```python
from build123d import *

# Parameters (mm, degrees)
F1_DEPTH = 5
F2_COUNT = 3
F3_DEPTH = 5


with BuildPart() as f1:
    # F0 (on Top) → F1 (new body)
    with BuildSketch(Plane.XY):
        with BuildLine():
            ThreePointArc((-5.4248477433, 6.6765403938), (0, 8.602625452), (5.4248477433, 6.6765403938))
            Line((5.4248477433, 6.6765403938), (1.3544146049, 29.8043473585))
            Line((1.3544146049, 29.8043473585), (-1.3544146049, 29.8043473585))
            Line((-1.3544146049, 29.8043473585), (-5.4248477433, 6.6765403938))
        make_face()
        with BuildLine():
            ThreePointArc((-6.4909440333, -0.3429949805), (-6.4880250922, 0.3943734303), (-6.4016109203, 1.1266665987))
            Line((-6.4016109203, 1.1266665987), (-6.5999012756, 0))
            Line((-6.5999012756, 0), (-6.4909440333, -0.3429949805))
        make_face()
        with BuildLine():
            ThreePointArc((-6.4016109203, 1.1266665987), (3.01e-08, 6.5), (6.4016109308, 1.1266665393))
            Line((6.4016109308, 1.1266665393), (5.4248477433, 6.6765403938))
            ThreePointArc((5.4248477433, 6.6765403938), (0, 8.602625452), (-5.4248477433, 6.6765403938))
            Line((-5.4248477433, 6.6765403938), (-6.4016109203, 1.1266665987))
        make_face()
        with BuildLine():
            ThreePointArc((5.4826146341, -20.6491084281), (3.2218551697, -19.3014479363), (0.6594098664, -18.7005351105))
            Line((0.6594098664, -18.7005351105), (0, -20.7763427347))
            Line((0, -20.7763427347), (-0.6594098664, -18.7005351105))
            ThreePointArc((-0.6594098664, -18.7005351105), (-3.2230425543, -19.3019277422), (-5.4845879123, -20.6507413875))
            Line((-5.4845879123, -20.6507413875), (-6.6083723171, -21.7710077677))
            ThreePointArc((-6.6083723171, -21.7710077677), (-8.5655271696, -26.4946509242), (-7.4957432876, -31.494533146))
            Line((-7.4957432876, -31.494533146), (-7.1801960351, -32.0117500748))
            ThreePointArc((-7.1801960351, -32.0117500748), (-4.7747668767, -34.4304254189), (-1.6183226323, -35.7238470784))
            ThreePointArc((-1.6183226323, -35.7238470784), (0, -35.7604840323), (1.6183226323, -35.7238470784))
            ThreePointArc((1.6183226323, -35.7238470784), (4.7779827917, -34.4282780127), (7.1844511071, -32.0052918853))
            Line((7.1844511071, -32.0052918853), (7.4957432876, -31.494533146))
            ThreePointArc((7.4957432876, -31.494533146), (8.3201892844, -29.4566518987), (8.6011218908, -27.2763427347))
            ThreePointArc((8.6011218908, -27.2763427347), (8.0881303689, -24.3503480465), (6.6103478907, -21.7733800287))
            Line((6.6103478907, -21.7733800287), (5.4826146341, -20.6491084281))
        make_face()
        with BuildLine():
            ThreePointArc((6.5, -27.2763427347), (-4.5961940777, -31.8725368124), (0, -20.7763427347))
            ThreePointArc((0, -20.7763427347), (4.5961940777, -22.680148657), (6.5, -27.2763427347))
        make_face(mode=Mode.SUBTRACT)
        with BuildLine():
            ThreePointArc((1.6183226323, -35.7238470784), (0, -35.7604840323), (-1.6183226323, -35.7238470784))
            ThreePointArc((-1.6183226323, -35.7238470784), (0, -35.8774646255), (1.6183226323, -35.7238470784))
        make_face()
        with BuildLine():
            Line((1.3493711691, -16.5285522429), (4.2182307974, -7.4974458056))
            ThreePointArc((4.2182307974, -7.4974458056), (0, -8.602625452), (-4.2182307974, -7.4974458056))
            Line((-4.2182307974, -7.4974458056), (-1.3493910102, -16.5284897836))
            Line((-1.3493910102, -16.5284897836), (0, -15.183323063))
            Line((0, -15.183323063), (1.3493711691, -16.5285522429))
        make_face()
        with BuildLine():
            Line((5.4248477433, 6.6765403938), (6.4016109308, 1.1266665393))
            Line((6.4016109308, 1.1266665393), (6.5999012756, 0))
            Line((6.5999012756, 0), (6.4909440333, -0.3429949805))
            ThreePointArc((6.4909440333, -0.3429949805), (6.1949432904, -1.9679119972), (5.498951298, -3.4657660946))
            Line((5.498951298, -3.4657660946), (4.2182307974, -7.4974458056))
            ThreePointArc((4.2182307974, -7.4974458056), (7.4260697643, -4.3426550086), (8.602625452, 0))
            ThreePointArc((8.602625452, 0), (7.7676604566, 3.6971091002), (5.4248477433, 6.6765403938))
        make_face()
        with BuildLine():
            Line((-6.5999012756, 0), (-6.4016109203, 1.1266665987))
            Line((-6.4016109203, 1.1266665987), (-5.4248477433, 6.6765403938))
            ThreePointArc((-5.4248477433, 6.6765403938), (-8.5716224911, -0.7296934543), (-4.2182307974, -7.4974458056))
            Line((-4.2182307974, -7.4974458056), (-5.498951298, -3.4657660946))
            ThreePointArc((-5.498951298, -3.4657660946), (-6.1949432904, -1.9679119972), (-6.4909440333, -0.3429949805))
            Line((-6.4909440333, -0.3429949805), (-6.5999012756, 0))
        make_face()
        with BuildLine():
            Line((0, -20.7763427347), (0.6594098664, -18.7005351105))
            ThreePointArc((0.6594098664, -18.7005351105), (0, -18.6752208439), (-0.6594098664, -18.7005351105))
            Line((-0.6594098664, -18.7005351105), (0, -20.7763427347))
        make_face()
        with BuildLine():
            Line((4.2182307974, -7.4974458056), (5.498951298, -3.4657660946))
            ThreePointArc((5.498951298, -3.4657660946), (0, -6.5), (-5.498951298, -3.4657660946))
            Line((-5.498951298, -3.4657660946), (-4.2182307974, -7.4974458056))
            ThreePointArc((-4.2182307974, -7.4974458056), (0, -8.602625452), (4.2182307974, -7.4974458056))
        make_face()
        with BuildLine():
            Line((0.6594098664, -18.7005351105), (1.3493711691, -16.5285522429))
            Line((1.3493711691, -16.5285522429), (0, -15.183323063))
            Line((0, -15.183323063), (-1.3493910102, -16.5284897836))
            Line((-1.3493910102, -16.5284897836), (-0.6594098664, -18.7005351105))
            ThreePointArc((-0.6594098664, -18.7005351105), (0, -18.6752208439), (0.6594098664, -18.7005351105))
        make_face()
        with BuildLine():
            Line((-0.6594098664, -18.7005351105), (-1.3493910102, -16.5284897836))
            Line((-1.3493910102, -16.5284897836), (-5.4845879123, -20.6507413875))
            ThreePointArc((-5.4845879123, -20.6507413875), (-3.2230425543, -19.3019277422), (-0.6594098664, -18.7005351105))
        make_face()
        with BuildLine():
            Line((5.4826146341, -20.6491084281), (1.3493711691, -16.5285522429))
            Line((1.3493711691, -16.5285522429), (0.6594098664, -18.7005351105))
            ThreePointArc((0.6594098664, -18.7005351105), (3.2218551697, -19.3014479363), (5.4826146341, -20.6491084281))
        make_face()
        with BuildLine():
            Line((-4.6210138798, 35.4606605825), (-1.3544146049, 29.8043473585))
            Line((-1.3544146049, 29.8043473585), (-0.3063812271, 35.7591715336))
            ThreePointArc((-0.3063812271, 35.7591715336), (-2.4682145028, 35.6752033686), (-4.6210138798, 35.4606605825))
        make_face()
        with BuildLine():
            Line((-1.3544146049, 29.8043473585), (1.3544146049, 29.8043473585))
            Line((1.3544146049, 29.8043473585), (0.3063812271, 35.7591715336))
            ThreePointArc((0.3063812271, 35.7591715336), (0, 35.7604840323), (-0.3063812271, 35.7591715336))
            Line((-0.3063812271, 35.7591715336), (-1.3544146049, 29.8043473585))
        make_face()
        with BuildLine():
            Line((0.3063812271, 35.7591715336), (1.3544146049, 29.8043473585))
            Line((1.3544146049, 29.8043473585), (4.6210138798, 35.4606605825))
            ThreePointArc((4.6210138798, 35.4606605825), (2.4682145028, 35.6752033686), (0.3063812271, 35.7591715336))
        make_face()
        with BuildLine():
            Line((-7.1801960351, -32.0117500748), (-5.1177123017, -35.3923895636))
            ThreePointArc((-5.1177123017, -35.3923895636), (-3.3720924779, -35.6011405793), (-1.6183226323, -35.7238470784))
            ThreePointArc((-1.6183226323, -35.7238470784), (-4.7747668767, -34.4304254189), (-7.1801960351, -32.0117500748))
        make_face()
        with BuildLine():
            ThreePointArc((1.6183226323, -35.7238470784), (3.3734184825, -35.601014957), (5.1203487512, -35.3920082348))
            Line((5.1203487512, -35.3920082348), (7.1844511071, -32.0052918853))
            ThreePointArc((7.1844511071, -32.0052918853), (4.7779827917, -34.4282780127), (1.6183226323, -35.7238470784))
        make_face()
    extrude(amount=F1_DEPTH)

    # F2: F1 ×3 about axis
    f2_axis = Axis((0, 0, 0), (0, 0, -1))


with BuildPart() as f1_1:
    add(f1.part)
    for i in range(1, F2_COUNT):
        add(f1.part.rotate(f2_axis, i * 360 / F2_COUNT))

    # F0 (on Top) → F3 (join)
    with BuildSketch(Plane.XY):
        with BuildLine():
            ThreePointArc((37.5, 0), (26.5165042945, 26.5165042945), (0, 37.5))
            ThreePointArc((0, 37.5), (-26.5165042945, -26.5165042945), (37.5, 0))
        make_face()
        with BuildLine():
            Line((0, 37.5), (0.3063812271, 35.7591715336))
            ThreePointArc((0.3063812271, 35.7591715336), (2.4682145028, 35.6752033686), (4.6210138798, 35.4606605825))
            ThreePointArc((4.6210138798, 35.4606605825), (26.8706337038, 23.5962128864), (35.7604840323, 0))
            ThreePointArc((35.7604840323, 0), (27.0362568413, -23.4062605778), (5.1203487512, -35.3920082348))
            ThreePointArc((5.1203487512, -35.3920082348), (3.3734184825, -35.601014957), (1.6183226323, -35.7238470784))
            ThreePointArc((1.6183226323, -35.7238470784), (0, -35.8774646255), (-1.6183226323, -35.7238470784))
            ThreePointArc((-1.6183226323, -35.7238470784), (-3.3720924779, -35.6011405793), (-5.1177123017, -35.3923895636))
            ThreePointArc((-5.1177123017, -35.3923895636), (-35.7596053622, 0.2506841909), (-4.6210138798, 35.4606605825))
            ThreePointArc((-4.6210138798, 35.4606605825), (-2.4682145028, 35.6752033686), (-0.3063812271, 35.7591715336))
            Line((-0.3063812271, 35.7591715336), (0, 37.5))
        make_face(mode=Mode.SUBTRACT)
        with BuildLine():
            ThreePointArc((-0.3063812271, 35.7591715336), (0, 35.7604840323), (0.3063812271, 35.7591715336))
            Line((0.3063812271, 35.7591715336), (0, 37.5))
            Line((0, 37.5), (-0.3063812271, 35.7591715336))
        make_face()
    extrude(amount=F3_DEPTH)


solid = f1_1.part
```
Here's how the part is built. I have some questions about the finished solid (model axes, mm). Give positions to 0.01 mm unless a question says otherwise; leave off trailing zeros. Write each loop counter-clockwise with the first axis right and the second up, starting at its lowest first coordinate (ties: lowest second). Pieces come first, ordered by that corner, then holes. Notation, with made-up numbers: (-17.5, 56.5) -> (27.5, 56.5) arc R15 ccw to (27.5, 60.5) -> close; hole circle Ø6 at (24.5, 56.5). An arc over 180 degrees is marked (long way). Use one line per item in the form item = value.
1) Suppose I cut it at A-A (y = 18). Please give me the cut outline in (x, z).
Verdict:
outline = (-32.9, 0) -> (-28.44, 0) -> (-28.44, 5) -> (-32.9, 5) -> close; (-18.8, 0) -> (-16.21, 0) -> (-16.21, 5) -> (-18.8, 5) -> close; (-3.43, 0) -> (3.43, 0) -> (3.43, 5) -> (-3.43, 5) -> close; (16.21, 0) -> (18.8, 0) -> (18.8, 5) -> (16.21, 5) -> close; (28.44, 0) -> (32.9, 0) -> (32.9, 5) -> (28.44, 5) -> close
2) If I drill on L1, parallel to Y at x = 0, z = 2; L2, parallel to X at y = -2.5, z = 3.55; L3, parallel to X at y = 17.5, z = 4.45, over which ranges is the centre line in solid material (lowest first)? Write a range as [from, to].
Verdict:
L1 = [-37.5, -33.78], [-20.78, -6.5], [6.5, 37.5]
L2 = [-37.42, -35.67], [-13.1, -6], [6, 13.1], [35.67, 37.42]
L3 = [-33.17, -28.85], [-18.39, -15.94], [-3.52, 3.52], [15.94, 18.39], [28.85, 33.17]
3) Suppose I cut it at B-B (z = 1.95). Give the number of separate pieces and of enclosed holes in the cut face, and give its area (3 significant figures).
Verdict:
separate_pieces = 1
enclosed_holes = 10
area = 1,520 mm2
4) We'd pull the mould along X, two halves only. Please class faces 1 (the face through (-6, -5, 0)), 2 (the face through (-3.28, 18.86, 2.46)), 3 (the face through (22.818, -29.759, 2.465)): +X half, -X half, draft (parallel to the pull), parting line (faces both ways), or undercut.
Verdict:
face_1 = draft
face_2 = undercut
face_3 = parting line
5) I'm going to push flat-ended pins straight in: pin 1 (10.5 mm diameter, centred on x = 23.62, y = 13.64, fed in from -Z); pin 2 (3 mm diameter, centred on x = 14, z = 3, fed in from +Y). Where does each tip first touch, or does it pass through?
Verdict:
pin_1 = through
pin_2 = 35.36
